from build123d import *

# Parameters (mm, degrees)
SKETCH2_R          = 49.53
SKETCH2_R_2        = 47.625
CUT_EXTRUDE1_DEPTH = 1.1176
CUT_EXTRUDE2_REACH = 107.371
SKETCH3_R          = 3.175


with BuildPart() as part:
    # Sketch1 → Revolve1 (revolve)
    with BuildSketch(Plane.XY):
        Polygon((0, 7.9375), (72.324156056, 50.8), (-20.347266862, 50.8), (-20.347266862, 69.85), (-33.047266862, 69.85), (-33.047266862, 50.8), (-33.047266862, 41.275), (-12.7, 7.9375), align=None)
    revolve(axis=Axis((0, 0, 0), (1, 0, 0)))

    # Sketch2 → Cut-Extrude1 (cut)
    with BuildSketch(Plane.ZY.offset(33.047266862)):
        Circle(SKETCH2_R)
        Circle(SKETCH2_R_2, mode=Mode.SUBTRACT)
    extrude(amount=-CUT_EXTRUDE1_DEPTH, mode=Mode.SUBTRACT)

    # Sketch3 → Cut-Extrude2 (cut, up to next)
    with BuildSketch(Plane.ZY.offset(33.047266862), mode=Mode.PRIVATE) as cut_extrude2_sk1:
        with Locations((0, 59.9186)):
            Circle(SKETCH3_R)
    cut_extrude2_tool1 = extrude(cut_extrude2_sk1.sketch, amount=-CUT_EXTRUDE2_REACH, mode=Mode.PRIVATE) & part.part
    add(cut_extrude2_tool1.solids().sort_by_distance((-33.047267, 59.9186, 0))[0], mode=Mode.SUBTRACT)
    # Sketch3 → Cut-Extrude2 (cut, up to next)
    with BuildSketch(Plane.ZY.offset(33.047266862), mode=Mode.PRIVATE) as cut_extrude2_sk2:
        with Locations((42.368848379, 42.368848379)):
            Circle(SKETCH3_R)
    cut_extrude2_tool2 = extrude(cut_extrude2_sk2.sketch, amount=-CUT_EXTRUDE2_REACH, mode=Mode.PRIVATE) & part.part
    add(cut_extrude2_tool2.solids().sort_by_distance((-33.047267, 42.368848, 42.368848))[0], mode=Mode.SUBTRACT)
    # Sketch3 → Cut-Extrude2 (cut, up to next)
    with BuildSketch(Plane.ZY.offset(33.047266862), mode=Mode.PRIVATE) as cut_extrude2_sk3:
        with Locations((59.9186, 0)):
            Circle(SKETCH3_R)
    cut_extrude2_tool3 = extrude(cut_extrude2_sk3.sketch, amount=-CUT_EXTRUDE2_REACH, mode=Mode.PRIVATE) & part.part
    add(cut_extrude2_tool3.solids().sort_by_distance((-33.047267, 0, 59.9186))[0], mode=Mode.SUBTRACT)
    # Sketch3 → Cut-Extrude2 (cut, up to next)
    with BuildSketch(Plane.ZY.offset(33.047266862), mode=Mode.PRIVATE) as cut_extrude2_sk4:
        with Locations((42.368848379, -42.368848379)):
            Circle(SKETCH3_R)
    cut_extrude2_tool4 = extrude(cut_extrude2_sk4.sketch, amount=-CUT_EXTRUDE2_REACH, mode=Mode.PRIVATE) & part.part
    add(cut_extrude2_tool4.solids().sort_by_distance((-33.047267, -42.368848, 42.368848))[0], mode=Mode.SUBTRACT)
    # Sketch3 → Cut-Extrude2 (cut, up to next)
    with BuildSketch(Plane.ZY.offset(33.047266862), mode=Mode.PRIVATE) as cut_extrude2_sk5:
        with Locations((0, -59.9186)):
            Circle(SKETCH3_R)
    cut_extrude2_tool5 = extrude(cut_extrude2_sk5.sketch, amount=-CUT_EXTRUDE2_REACH, mode=Mode.PRIVATE) & part.part
    add(cut_extrude2_tool5.solids().sort_by_distance((-33.047267, -59.9186, 0))[0], mode=Mode.SUBTRACT)
    # Sketch3 → Cut-Extrude2 (cut, up to next)
    with BuildSketch(Plane.ZY.offset(33.047266862), mode=Mode.PRIVATE) as cut_extrude2_sk6:
        with Locations((-42.368848379, -42.368848379)):
            Circle(SKETCH3_R)
    cut_extrude2_tool6 = extrude(cut_extrude2_sk6.sketch, amount=-CUT_EXTRUDE2_REACH, mode=Mode.PRIVATE) & part.part
    add(cut_extrude2_tool6.solids().sort_by_distance((-33.047267, -42.368848, -42.368848))[0], mode=Mode.SUBTRACT)
    # Sketch3 → Cut-Extrude2 (cut, up to next)
    with BuildSketch(Plane.ZY.offset(33.047266862), mode=Mode.PRIVATE) as cut_extrude2_sk7:
        with Locations((-59.9186, 0)):
            Circle(SKETCH3_R)
    cut_extrude2_tool7 = extrude(cut_extrude2_sk7.sketch, amount=-CUT_EXTRUDE2_REACH, mode=Mode.PRIVATE) & part.part
    add(cut_extrude2_tool7.solids().sort_by_distance((-33.047267, 0, -59.9186))[0], mode=Mode.SUBTRACT)
    # Sketch3 → Cut-Extrude2 (cut, up to next)
    with BuildSketch(Plane.ZY.offset(33.047266862), mode=Mode.PRIVATE) as cut_extrude2_sk8:
        with Locations((-42.368848379, 42.368848379)):
            Circle(SKETCH3_R)
    cut_extrude2_tool8 = extrude(cut_extrude2_sk8.sketch, amount=-CUT_EXTRUDE2_REACH, mode=Mode.PRIVATE) & part.part
    add(cut_extrude2_tool8.solids().sort_by_distance((-33.047267, 42.368848, -42.368848))[0], mode=Mode.SUBTRACT)


solid = part.part
Could you check a few things on this model? Use its own coordinates, in mm. A direction names the side the tool comes from. Round coordinates to 2 decimals unless told otherwise and drop trailing zeros. Write each loop counter-clockwise with the first axis right and the second up, starting at its lowest first coordinate (ties: lowest second). Pieces come first, ordered by that corner, then holes. Notation, with made-up numbers: (41.25, 23.5) -> (58.25, 23.5) arc R20 cw to (58.25, 49.5) -> close; hole circle Ø9 at (71.25, 79.5). An arc over 180 degrees is marked (long way). Use a Markdown table: item, result.
1. For pin 1 Ø10 at (y, z) = (42.37, -42.37) entering from +X; pin 2 Ø2 at (y, z) = (15, -35) entering from -X; pin 3 Ø8 at (x, z) = (52.5, -8.5) entering from -Y; pin 4 Ø10 at (y, z) = (59.92, 0) entering from -X, each with a flat end and sliding along its axis, tell me the tip position at first contact or that it passes through.
Answer key:
| item | result |
|---|---|
| pin 1 | stops at x = -20.35 |
| pin 2 | stops at x = -31.71 |
| pin 3 | stops at y = -50.6 |
| pin 4 | stops at x = -33.05 |
2. We'd pull the mould along Z, two halves only. Please class faces 1 (the face through (-33.047, -14, 39)), 2 (the face through (20.6, 19.2, 6.1)), 3 (the face through (25.34, -11.012, -49.592)): +Z half, -Z half, draft (parallel to the pull), parting line (faces both ways), or undercut.
Answer key:
| item | result |
|---|---|
| face 1 | draft |
| face 2 | undercut |
| face 3 | parting line |
3. If we section it at C-C (x = -2.5): List the corners of the cut face in (y, z) for me (1 decimal).
Answer key:
| item | result |
|---|---|
| outline | circle Ø101.6 at (0, 0); hole circle Ø15.9 at (0, 0) |
4. Which directions (+Z, -Z, +X, -X, +Y, -Y) give clear straight access to the entire face, cutting with the end or side of a thin tool? Please do faces 4 (the face through (-26.786, 44.515, -44.709)), 5 (the face through (-20.347, -31, -41)), 6 (the face through (-31.93, 41, -26)).
Answer key:
| item | result |
|---|---|
| face 4 | +X, -X |
| face 5 | +X |
| face 6 | -X |
5. If we section it at A-A (z = 0): State how many separate pieces and enclosed holes the cut face has, then the cut area to 3 significant figures.
Answer key:
| item | result |
|---|---|
| separate pieces | 4 |
| enclosed holes | 0 |
| area | 5,570 mm^2 |
6. If we section it at D-D (x = 37): List the corners of the cut face in (y, z) for me.
Answer key:
| item | result |
|---|---|
| outline | circle Ø101.6 at (0, 0); hole circle Ø59.73 at (0, 0) |
7. Please list where these lines run through material, in increasing order: probe 1 along Z at (x, y) = (-5.25, 0); probe 2 along Y at (x, z) = (-5.5, 6); probe 3 along Z at (x, y) = (51, 18.5).
Answer key:
| item | result |
|---|---|
| probe 1 | z = -50.8 to -7.94, 7.94 to 50.8 |
| probe 2 | y = -50.44 to -5.2, 5.2 to 50.44 |
| probe 3 | z = -47.31 to -33.38, 33.38 to 47.31 |
